The figure shows three views and two pictorial views of one solid part (mm, origin at its lowest corner). Answer the questions. A direction names the side the tool comes from. Give positions to 0.01 mm unless a question says otherwise; leave off trailing zeros. Loops run counter-clockwise (first coordinate to the right, second up) from the corner with the lowest first, then second, coordinate; pieces in that order, holes last. Notation, with made-up numbers: M 83,-0.5 L 132,-0.5 A28 ccw 132,38.5 Z; hole C 5.5,-35 d11. An arc over 180 degrees is marked long. Write item = value, one per line. Start each with the question number.
1. Consider L1, parallel to Y at x = 2.5, z = 120.5; L2, parallel to Z at x = 7.5, y = 127; L3, parallel to Z at x = 20, y = 103.5. Determine where each line is inside the solid, lowest interval first. Write a range as [from, to].
2. Section A-A on x = 5 is taken. Determine the outline of the cut face in (y, z), plus the area to 3 significant figures.
3. For the marked faces 1 and 2, determine the directions among +Z, -Z, +X, -X, +Y, -Y from which every point of the face is accessible in a straight line to the end or side of a thin tool.
4. The mould has two halves that part along Z. Classify the marked faces 3, 4 and 5: released by +Z, released by -Z, zero draft, split by the parting line, or undercut.
5. Section C-C on y = 122 is taken. Determine the outline of the cut face in (x, z), plus the area to 3 significant figures.
6. Section B-B on z = 156.5 is taken. Determine the outline of the cut face in (x, y), plus the area to 3 significant figures.
7. Flat-ended cylindrical pins translate along their axes: pin 1 Ø1 at (x, z) = (16.5, 151) entering from -Y; pin 2 Ø10 at (x, y) = (14.5, 15) entering from -Z; pin 3 Ø2 at (x, z) = (19, 224.5) entering from +Y. Find the tip coordinate at first contact, or state that the pin passes through.
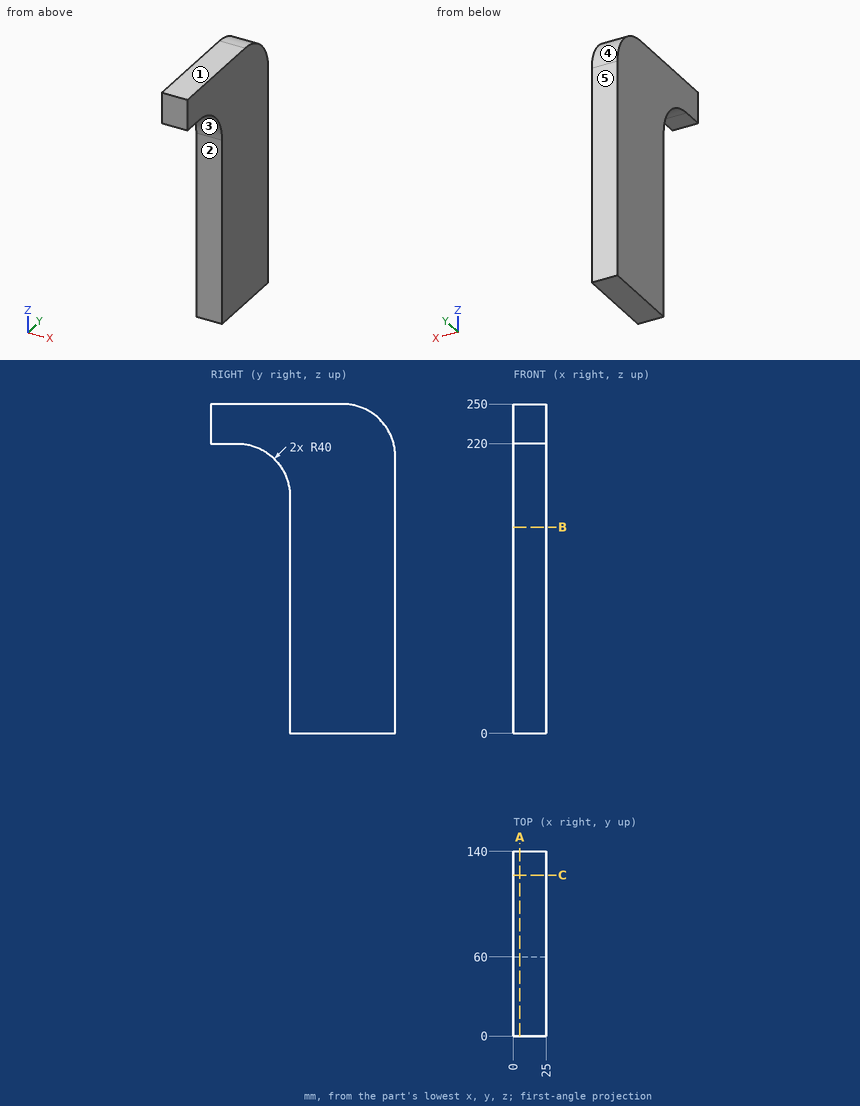
Verdict:
q1.L1 = [60, 140]
q1.L2 = [0, 239.51]
q1.L3 = [0, 249.85]
q2.outline = M 0,220 L 20,220 A40 cw 60,180 L 60,0 L 140,0 L 140,210 A40 ccw 100,250 L 0,250 Z
q2.area = 21,800 mm2
q3.face_1 = +Z, +X, -X, +Y, -Y
q3.face_2 = -Z, +X, -X, -Y
q4.face_3 = released by -Z
q4.face_4 = released by +Z
q4.face_5 = zero draft
q5.outline = M 0,0 L 25,0 L 25,243.41 L 0,243.41 Z
q5.area = 6,090 mm2
q6.outline = M 0,60 L 25,60 L 25,140 L 0,140 Z
q6.area = 2,000 mm2
q7.pin_1 = 60
q7.pin_2 = 220
q7.pin_3 = 137.65
